Here's how the part is built. I have some questions about the finished solid (model axes, mm). A direction names the side the tool comes from. Give positions to 0.01 mm unless a question says otherwise; leave off trailing zeros. Write each loop counter-clockwise with the first axis right and the second up, starting at its lowest first coordinate (ties: lowest second). Pieces come first, ordered by that corner, then holes. Notation, with made-up numbers: (41, -8.5) -> (56, -8.5) arc R7 ccw to (56, -0.5) -> close; hole circle Ø3 at (22.5, 65). An arc over 180 degrees is marked (long way). Use one line per item in the form item = value.
```python
from build123d import *

# Parameters (mm, degrees)
EXTRUDE_1_DEPTH = 70


with BuildPart() as part:
    # 草图1 → 凸台-拉伸1 (new body)
    with BuildSketch(Plane(origin=(0, 0, 0), x_dir=(1, 0, 0), z_dir=(0, 1, 0))):
        Polygon((-1226.000639084, 113.615915427), (1103.964935241, 113.615915427), (1043.964935241, 32.273003651), (843.964935241, 32.273003651), (843.964935241, -167.726996349), (783.964935241, -246.384084573), (-906.000639084, -246.384084573), (-965.035064759, -167.726996349), (-965.035064759, 32.273003651), (-1166.000639084, 32.273003651), align=None)
    extrude(amount=EXTRUDE_1_DEPTH)


solid = part.part
```
Q1. If we mould it in two halves opening along Z, with no side actions, what happens to faces 1 (the face through (-45, 70, 64)), 2 (the face through (814.385, 34.51, 206.505)), 3 (the face through (-77, 35, -113.616))? For each: +Z half, -Z half, draft (parallel to the pull), parting line (faces both ways), or undercut.
Result set:
face_1 = draft
face_2 = +Z half
face_3 = -Z half
Q2. If I drill on line 1 along Z through (x, y) = (-985.5, 56); line 2 along X through (y, z) = (54, 146); line 3 along X through (y, z) = (7, 213), over which ranges is the centre line in solid material (lowest first)? Write a range as from..to.
Result set:
line_1 = -113.62..-32.27
line_2 = -965.04..843.96
line_3 = -931.06..809.43
Q3. Will these pins go through, and if not, where does the flat tip stop? pin 1 Ø21 at (x, y) = (989, 22) entering from +Z; pin 2 Ø4 at (y, z) = (30.5, -63) entering from +X; pin 3 Ø3 at (y, z) = (26, 45.5) entering from +X.
Result set:
pin_1 = -32.27
pin_2 = 1068.1
pin_3 = 843.96
Q4. Which directions (+Z, -Z, +X, -X, +Y, -Y) give clear straight access to the entire face, cutting with the end or side of a thin tool? Please do faces 4 (the face through (-965.035, 35, 69)), 5 (the face through (843.965, 35, 66)), 6 (the face through (-49, 35, 246.384)).
Result set:
face_4 = +Z, -X, +Y, -Y
face_5 = +Z, +X, +Y, -Y
face_6 = +Z, +X, -X, +Y, -Y
Q5. I want a section at A-A, the plane y = 46.5. Write out the boundary of the cut face in (x, z).
Result set:
outline = (-1226, -113.62) -> (1103.96, -113.62) -> (1043.96, -32.27) -> (843.96, -32.27) -> (843.96, 167.73) -> (783.96, 246.38) -> (-906, 246.38) -> (-965.04, 167.73) -> (-965.04, -32.27) -> (-1166, -32.27) -> close
Q6. I want a section at B-B, the plane z = 45. Write out the boundary of the cut face in (x, y).
Result set:
outline = (-965.04, 0) -> (843.96, 0) -> (843.96, 70) -> (-965.04, 70) -> close
